```python
from build123d import *

# Parameters (mm, degrees)
BOSS_EXTRUDE1_DEPTH = 12
CUT_EXTRUDE1_DEPTH  = 10
SKETCH3_R           = 2.5
SKETCH3_R_2         = 1.5
BOSS_EXTRUDE2_DEPTH = 1.2
SKETCH4_R           = 2.5
BOSS_EXTRUDE3_DEPTH = 5
CHAMFER1_SIZE       = 0.5


with BuildPart() as part:
    # Sketch1 → Boss-Extrude1 (new body)
    with BuildSketch(Plane(origin=(0, 0, 0), x_dir=(1, 0, 0), z_dir=(0, 1, 0))):
        with BuildLine():
            Line((-23.25, -5), (-5.749755012, -5))
            Line((-5.749755012, -5), (-5.749755012, 0))
            add(Edge.make_bspline(
                [(-3.25, 5), (-5.749755012, 5), (-5.749755012, 0)],
                knots=[0, 0, 0, 1.570796327, 1.570796327, 1.570796327], degree=2, weights=[1, 0.707106781, 1]))
            Line((-3.25, 5), (3.25, 5))
            add(Edge.make_bspline(
                [(5.748694825, 0), (5.748694825, 5), (3.25, 5)],
                knots=[4.71238898, 4.71238898, 4.71238898, 6.283185307, 6.283185307, 6.283185307], degree=2, weights=[1, 0.707106781, 1]))
            Line((5.748694825, 0), (5.748694825, -5))
            Line((5.748694825, -5), (23.25, -5))
            Line((23.25, -5), (23.25, -3))
            Line((23.25, -3), (9.282157642, -3))
            ThreePointArc((9.282157642, -3), (8.511424396, -2.637157958), (8.3, -1.811940526))
            Line((8.3, -1.811940526), (8.3, 6.6))
            Line((8.3, 6.6), (-8.3, 6.6))
            Line((-8.3, 6.6), (-8.3, -1.812055437))
            ThreePointArc((-8.3, -1.812055437), (-8.511483666, -2.637203044), (-9.282179638, -3))
            Line((-9.282179638, -3), (-23.25, -3))
            Line((-23.25, -3), (-23.25, -5))
        make_face()
    extrude(amount=BOSS_EXTRUDE1_DEPTH)

    # Sketch2 → Cut-Extrude1 (cut)
    with BuildSketch(Plane(origin=(0, 0, 3), x_dir=(-1, 0, 0), z_dir=(0, 0, -1))):
        Polygon((19.85850269, 6), (18.068716856, 9.1), (14.489145187, 9.1), (12.699359352, 6), (14.489145187, 2.9), (18.068716856, 2.9), align=None)
        Polygon((-12.686507152, 6), (-14.476292987, 9.1), (-18.055864656, 9.1), (-19.84565049, 6), (-18.055864656, 2.9), (-14.476292987, 2.9), align=None)
    extrude(amount=-CUT_EXTRUDE1_DEPTH, mode=Mode.SUBTRACT)

    # Sketch3 → Boss-Extrude2 (add)
    with BuildSketch(Plane(origin=(0, 12, 0), x_dir=(1, 0, 0), z_dir=(0, 1, 0))):
        with BuildLine():
            Line((-8.3, 6.6), (8.3, 6.6))
            Line((8.3, 6.6), (8.3, 10.6))
            ThreePointArc((8.3, 10.6), (0, 13.462912018), (-8.3, 10.6))
            Line((-8.3, 10.6), (-8.3, 6.6))
        make_face()
        with Locations(Location((-3.25, 9.48526903, 0), (0, 0, 270))):
            Circle(SKETCH3_R, mode=Mode.SUBTRACT)
        with Locations(Location((3.25, 9.48526903, 0), (0, 0, 270))):
            Circle(SKETCH3_R_2, mode=Mode.SUBTRACT)
    extrude(amount=-BOSS_EXTRUDE2_DEPTH)

    # Sketch4 → Boss-Extrude3 (add)
    with BuildSketch(Plane.XZ.offset(-10.8)):
        with BuildLine():
            Line((8.3, -6.6), (-8.3, -6.6))
            Line((-8.3, -6.6), (-8.3, -10.6))
            ThreePointArc((-8.3, -10.6), (0, -13.462912018), (8.3, -10.6))
            Line((8.3, -10.6), (8.3, -6.6))
        make_face()
        with Locations(Location((-3.25, -9.48526903, 0), (0, 0, 90))):
            Circle(SKETCH4_R, mode=Mode.SUBTRACT)
        with Locations(Location((3.25, -9.48526903, 0), (0, 0, 270))):
            Circle(SKETCH4_R, mode=Mode.SUBTRACT)
    extrude(amount=BOSS_EXTRUDE3_DEPTH)

    # Chamfer1
    chamfer1_edges = [part.edges().sort_by_distance(p)[0] for p in [
        (0, 12, -5),
        (-5.260112096, 12, -2.972310439),
        (5.259369228, 12, -2.972013605),
        (-5.749755012, 12, 2.5),
        (5.748694825, 12, 2.5),
    ]]
    chamfer(chamfer1_edges, length=CHAMFER1_SIZE)


solid = part.part
```
Source: CAD feature listing. Evaluate the final solid. Frame: model axes, mm. A direction names the side the tool comes from. Give positions to 0.01 mm unless a question says otherwise; leave off trailing zeros. Loops run counter-clockwise (first coordinate to the right, second up) from the corner with the lowest first, then second, coordinate; pieces in that order, holes last. Notation, with made-up numbers: (-10, 43.25) - (39, 43.25) arc R23 ccw to (39, 75.25) - close; hole circle Ø3 at (32.5, 73.5). An arc over 180 degrees is marked (long way). Use CSV: the item, a comma, the result in double quotes.
1) Pin query (flat end, axial travel): P1, Ø4.5, axis at x = 0.5, y = 3, coming from the -Z side; P2, Ø5, axis at y = 6, z = -0.5, coming from the -X side; P3, Ø4, axis at x = 3.25, z = -9.49, coming from the +Y side; P4, Ø2, axis at y = 5, z = 1.5, coming from the +X side. Return the tip coordinate at first contact, or that it passes through.
Worked out:
P1,"stops at z = -6.6"
P2,"stops at x = -8.3"
P3,"stops at y = 12"
P4,"stops at x = 8.42"
2) Line query: line 1 (X direction, y = 6, z = -11.5); line 2 (X direction, y = 9.5, z = 3.75); line 3 (Z direction, x = -6.5, y = 1.75). Output: solid intervals per line, ascending.
Worked out:
line 1,"x = -7 to -4.73, -1.77 to 1.77, 4.73 to 7"
line 2,"x = -23.25 to -5.75, 5.75 to 23.25"
line 3,"z = -6.6 to 5"
3) Cut plane A-A (z = 2.25). Output: boundary loops of the cut face in (x, y), and give its area (3 significant figures).
Worked out:
outline,"(-8.31, 0) - (-5.75, 0) - (-5.75, 11.5) - (-6.25, 12) - (-8.31, 12) - close; (5.75, 0) - (8.31, 0) - (8.31, 12) - (6.25, 12) - (5.75, 11.5) - close"
area,"61.3 mm^2"
4) Mould query, pull axis Y, two halves, no side actions, for faces 4 (the flat face through (4, 10.8, -8)), 5 (the flat face through (16, 2.9, 4)), 6 (the flat face through (-13, 5, 5)). Classes: +Y half, -Y half, draft (parallel to the pull), parting line (faces both ways), or undercut.
Worked out:
face 4,"-Y half"
face 5,"undercut"
face 6,"draft"
5) Cut plane B-B (z = -8.5). Output: boundary loops of the cut face in (x, y), and give its area (3 significant figures).
Worked out:
outline,"(-8.3, 5.8) - (-5.55, 5.8) - (-5.55, 12) - (-8.3, 12) - close; (-0.95, 5.8) - (0.95, 5.8) - (0.95, 10.8) - (2.12, 10.8) - (2.12, 12) - (-0.95, 12) - close; (4.38, 10.8) - (5.55, 10.8) - (5.55, 5.8) - (8.3, 5.8) - (8.3, 12) - (4.38, 12) - close"
area,"48.7 mm^2"
6) Cut plane C-C (y = 7.5). Count the separate pieces of the cut face and the enclosed holes in it, and give its area (3 significant figures).
Worked out:
separate pieces,"3"
enclosed holes,"2"
area,"181 mm^2"
7) Cut plane D-D (x = 7). Output: boundary loops of the cut face in (y, z).
Worked out:
outline,"(0, -6.6) - (5.8, -6.6) - (5.8, -11.5) - (12, -11.5) - (12, 5) - (0, 5) - close"
8) Set-up query: faces 1 (the flat face through (16, 9.1, 4)), 2 (the flat face through (-5.75, 6, 3)), 3 (the flat face through (19.5, 4.6, 3)). Return all of +Z, -Z, +X, -X, +Y, -Y with unobstructed straight access to the full face (end or side cutting, diameter ignored); none if empty.
Worked out:
face 1,"+Z, -Z"
face 2,"+Z, +Y, -Y"
face 3,"-Z, +X, +Y, -Y"
